Geometry: final body of the model. Coordinates: model frame, mm. A direction names the side the tool comes from. Coordinates: 2 decimals unless noted, no trailing zeros. Loops run counter-clockwise (first coordinate to the right, second up) from the corner with the lowest first, then second, coordinate; pieces in that order, holes last. Notation, with made-up numbers: (47, 32) -> (61, 32) arc R10 ccw to (61, 43) -> close; hole circle Ø7 at (0.5, 89). An arc over 180 degrees is marked (long way). One line per item, written item: value. Start each with the question number.
Item 1: Section query C-C on z = 3.25. Return loops of the section in (x, y), then the cut area to 3 significant figures.
Item 2: Mould query, pull axis X, two halves, no side actions, for faces 3 (the flat face through (9, -9, 0)), 4 (the cylindrical face through (-4.336, 19.524, 4.93)), 5 (the cylindrical face through (-17, 0, 5)). Classes: +X half, -X half, draft (parallel to the pull), parting line (faces both ways), or undercut.
Item 3: Contact query for flat-ended pins moving along their axis: pin 1 Ø3 at (x, z) = (-3, -9) entering from +Y; pin 2 Ø8 at (y, z) = (10.5, 0) entering from +X; pin 3 Ø1.5 at (x, z) = (6.5, -7) entering from +Y. Output: stop coordinate, or through.
Item 4: Section query D-D on y = -8.5. Return loops of the section in (x, z).
Item 5: Section query A-A on x = 0. Return loops of the section in (y, z), then the cut area to 3 significant figures.
Item 6: Ray query, probe 1 along Y at (x, z) = (0, 4.75); probe 2 along X at (y, z) = (0.5, 2.25); probe 3 along X at (y, z) = (14, 7.25). Return the intervals inside material, ascending. Write a range as from..to.
Item 7: Section query B-B on y = 0. Return loops of the section in (x, z), then the cut area to 3 significant figures.
Item 8: Set-up query: faces 1 (the cylindrical face through (1.2, -15.6, 5.1)), 2 (the cylindrical face through (-1.5, 11.4, -5.9)). Return all of +Z, -Z, +X, -X, +Y, -Y with unobstructed straight access to the full face (end or side cutting, diameter ignored); none if empty.
Autodesk Fusion 360 part; units mm, degrees
sketch "Sketch1" plane through (0, 0, 0) normal (0, 0, 1) x (1, 0, 0)
  circle A0 centre (0, 0) radius 20
  circle A1 centre (0, 0) radius 4
  circle A2 centre (0, 0) radius 11.5
  point P0 (-15, 0)
  point P1 (15, 0)
  point P2 (0, 14)
  point P3 (0, -14)
  dimension "d1" = 40
  dimension "d2" = 8
  dimension "d3" = 15
  dimension "d4" = 15
  dimension "d5" = 14
  dimension "d6" = 14
  dimension "d7" = 23
extrude "Extrude1" add sketch "Sketch1" along normal blind 10 contours A0 | A2
extrude "Extrude2" add sketch "Sketch1" against normal blind 12 contours A2
hole "Hole1" at (0, 14, 0) at (15, 0, 0) at (0, -14, 0) at (-15, 0, 0) direction (0, 0, 1) diameter 4 depth 20 tip angle 118
ref_plane "WorkPlane1" through (8.1317, 8.1317, -4.9786) normal (0.7071, 0.7071, 0) x (-0.7071, 0.7071, 0)
hole "Hole2" at (7.9968, 8.2666, -5.7724) direction (-0.7071, -0.7071, 0) diameter 4 depth 12 tip angle 118
Reply:
1. outline: circle Ø40 at (0, 0); hole circle Ø4 at (-15, 0); hole circle Ø8 at (0, 0); hole circle Ø4 at (0, -14); hole circle Ø4 at (0, 14); hole circle Ø4 at (15, 0)
1. area: 1,160 mm²
2. face 3: draft
2. face 4: parting line
2. face 5: undercut
3. pin 1: stops at y = 11.4
3. pin 2: stops at x = 18.91
3. pin 3: stops at y = 9.96
4. outline: (-18.1, 0) -> (-7.75, 0) -> (-7.75, -12) -> (7.75, -12) -> (7.75, 0) -> (18.1, 0) -> (18.1, 10) -> (-18.1, 10) -> close
5. outline: (-20, 0) -> (-16, 0) -> (-16, 10) -> (-20, 10) -> close; (-12, 0) -> (-11.5, 0) -> (-11.5, -12) -> (-4, -12) -> (-4, 10) -> (-12, 10) -> close; (4, -12) -> (11.5, -12) -> (11.5, 0) -> (12, 0) -> (12, 10) -> (4, 10) -> close; (16, 0) -> (20, 0) -> (20, 10) -> (16, 10) -> close
5. area: 420 mm²
6. probe 1: y = -20..-16, -12..-4, 4..12, 16..20
6. probe 2: x = -19.99..-16.94, -13.06..-3.97, 3.97..13.06, 16.94..19.99
6. probe 3: x = -14.28..-2, 2..14.28
7. outline: (-20, 0) -> (-17, 0) -> (-17, 10) -> (-20, 10) -> close; (-13, 0) -> (-11.5, 0) -> (-11.5, -12) -> (-4, -12) -> (-4, 10) -> (-13, 10) -> close; (4, -12) -> (11.5, -12) -> (11.5, 0) -> (13, 0) -> (13, 10) -> (4, 10) -> close; (17, 0) -> (20, 0) -> (20, 10) -> (17, 10) -> close
7. area: 420 mm²
8. face 1: +Z, -Z
8. face 2: -Z
